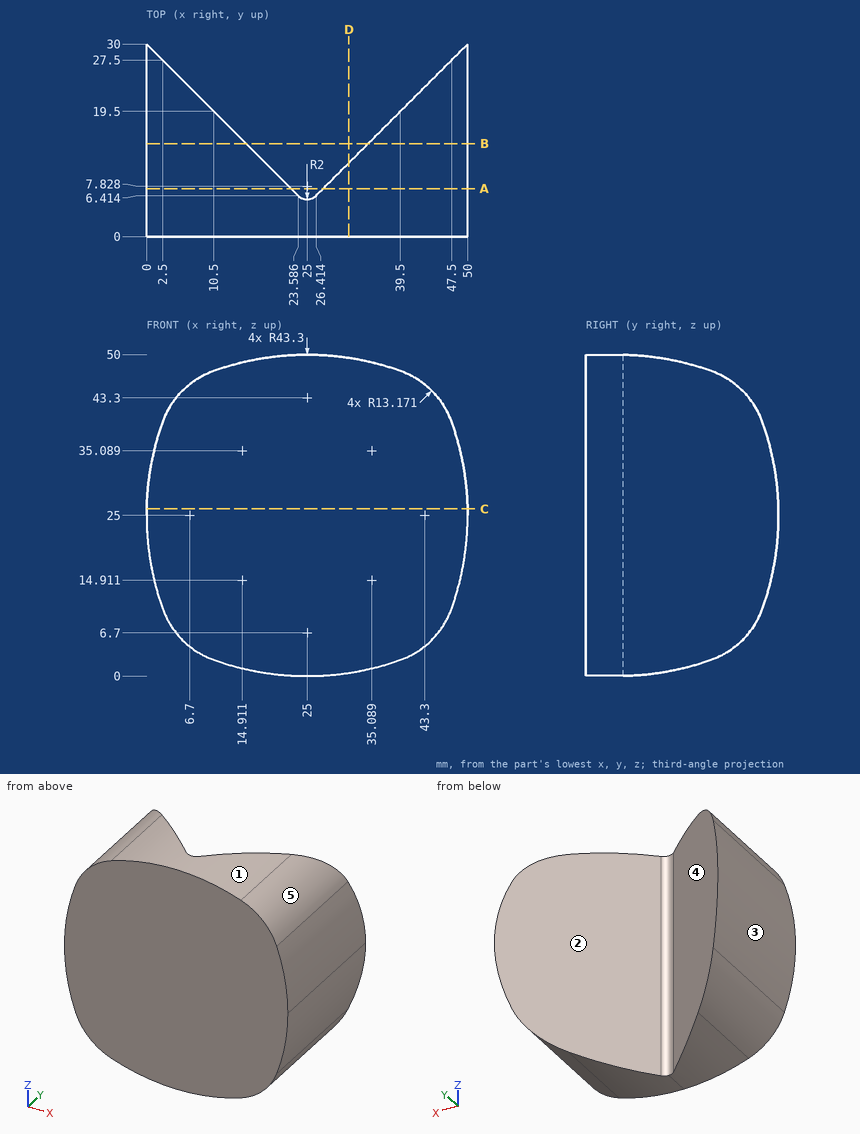
For this review, use the dimensioned drawing (mm, ordinates from the lowest corner) and the shaded views. A direction names the side the tool comes from. Round coordinates to 2 decimals unless told otherwise and drop trailing zeros. Write each loop counter-clockwise with the first axis right and the second up, starting at its lowest first coordinate (ties: lowest second). Pieces come first, ordered by that corner, then holes. Notation, with made-up numbers: (14.5, 49.25) - (21.5, 49.25) arc R26 ccw to (21.5, 74.25) - close; hole circle Ø11 at (-10.75, 14). An arc over 180 degrees is marked (long way). Answer as CSV lines item,"result". Start each with the question number.
(1) We need section D-D on x = 31.5. State the section outline as (y, z) points.
(2) To check wall thickness, follow line 1 (X direction, y = 20, z = 32.5) (1 decimal); line 2 (X direction, y = 9, z = 26); line 3 (Y direction, x = 15, z = 41.5). State the ranges of each line that lie inside material, in increasing order.
(3) We need section C-C on z = 26. State the section outline as (x, y) points (1 decimal).
(4) We need section B-B on y = 14.5. State the section outline as (x, z) points (1 decimal).
(5) For the marked faces 1 and 2, list the 3-axis set-ups (+Z, -Z, +X, -X, +Y, -Y) from which the entire face can be reached by the end or side of a thin tool; tool diameter is ignored.
(6) Draft analysis for pull direction X (two halves, no side actions). For the marked faces 3, 4 and 5, state which applies: pulls with the +X half, pulls with the -X half, needs draft (parallel to the pull), parting line crosses it, or undercut.
(7) For pin 1 Ø12 at (y, z) = (17, 37) entering from +X; pin 2 Ø10 at (y, z) = (16.5, 9) entering from -X; pin 3 Ø5 at (x, z) = (32, 37) entering from +Y, all flat-tipped, find the tip position at first contact; note any pin that passes through.
(8) We need section A-A on y = 7.5. State the section outline as (x, z) points, plus the area to 3 significant figures.
Worked answers:
1,outline,"(0, 0.49) - (11.5, 0.49) - (11.5, 49.51) - (0, 49.51) - close"
2,line 1,"0.7 to 10, 40 to 49.3"
2,line 2,"0.01 to 21, 29 to 49.99"
2,line 3,"0 to 15"
3,outline,"(0, 0) - (50, 0) - (50, 30) - (26.4, 6.4) arc R2 cw to (23.6, 6.4) - (0, 30) - close"
4,outline,"(2.5, 10.5) arc R13.2 ccw to (10.5, 2.5) arc R43.3 ccw to (15.5, 1.1) - (15.5, 48.9) arc R43.3 ccw to (10.5, 47.5) arc R13.2 ccw to (2.5, 39.5) arc R43.3 ccw to start; (34.5, 1.1) arc R43.3 ccw to (39.5, 2.5) arc R13.2 ccw to (47.5, 10.5) arc R43.3 ccw to (47.5, 39.5) arc R13.2 ccw to (39.5, 47.5) arc R43.3 ccw to (34.5, 48.9) - close"
5,face 1,"+Z, +Y, -Y"
5,face 2,"+Z, -Z, +Y"
6,face 3,"pulls with the -X half"
6,face 4,"undercut"
6,face 5,"pulls with the +X half"
7,pin 1,"x = 49.58"
7,pin 2,"x = 1.42"
7,pin 3,"y = 14.5"
8,outline,"(2.5, 10.5) arc R13.17 ccw to (10.5, 2.5) arc R43.3 ccw to (22.5, 0.07) - (22.5, 49.93) arc R43.3 ccw to (10.5, 47.5) arc R13.17 ccw to (2.5, 39.5) arc R43.3 ccw to start; (27.5, 0.07) arc R43.3 ccw to (39.5, 2.5) arc R13.17 ccw to (47.5, 10.5) arc R43.3 ccw to (47.5, 39.5) arc R13.17 ccw to (39.5, 47.5) arc R43.3 ccw to (27.5, 49.93) - close"
8,area,"1,880 mm²"
